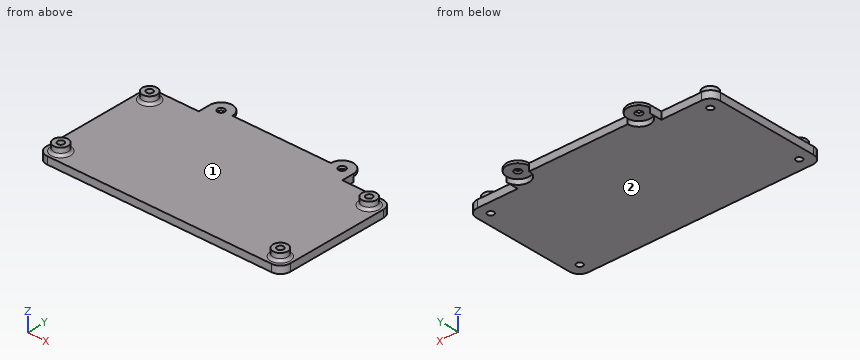
from build123d import *

# Parameters (mm, degrees)
SKETCH1_R           = 3
BOSS_EXTRUDE1_DEPTH = 3
SKETCH1_3_R         = 3
SKETCH1_3_R_2       = 1.3
BOSS_EXTRUDE2_DEPTH = 6
FILLET1_R           = 1
SKETCH2_R           = 1.4224
BOSS_EXTRUDE3_DEPTH = 3
CUT_EXTRUDE1_START  = -2
SKETCH6_R           = 4.618405104
CUT_EXTRUDE1_DEPTH  = 2


with BuildPart() as part:
    # Sketch1 → Boss-Extrude1 (new body)
    with BuildSketch(Plane.XY):
        with BuildLine():
            ThreePointArc((99.987500635, 4.00000762), (98.819645279, 1.180555381), (96.00019304, 0.012700025))
            Line((96.00019304, 0.012700025), (4.00000762, 0.012700025))
            ThreePointArc((4.00000762, 0.012700025), (1.180555381, 1.180555381), (0.012700025, 4.00000762))
            Line((0.012700025, 4.00000762), (0.012700025, 46.00009144))
            ThreePointArc((0.012700025, 46.00009144), (1.180555381, 48.819543679), (4.00000762, 49.987399035))
            Line((4.00000762, 49.987399035), (96.00019304, 49.987399035))
            ThreePointArc((96.00019304, 49.987399035), (98.819645279, 48.819543679), (99.987500635, 46.00009144))
            Line((99.987500635, 46.00009144), (99.987500635, 4.00000762))
        make_face()
        with Locations((95.0001905, 5.00001016)):
            Circle(SKETCH1_R, mode=Mode.SUBTRACT)
        with Locations((5.00001016, 5.00001016)):
            Circle(SKETCH1_R, mode=Mode.SUBTRACT)
        with Locations((95.0001905, 45.0000889)):
            Circle(SKETCH1_R, mode=Mode.SUBTRACT)
        with Locations((5.00001016, 45.0000889)):
            Circle(SKETCH1_R, mode=Mode.SUBTRACT)
    extrude(amount=BOSS_EXTRUDE1_DEPTH)

    # Sketch1<3> → Boss-Extrude2 (add)
    # profile 1 of 4: a face of its own
    with BuildSketch(Plane.XY):
        with Locations((5.00001016, 45.0000889)):
            Circle(SKETCH1_3_R)
        with Locations((5.00001016, 45.0000889)):
            Circle(SKETCH1_3_R_2, mode=Mode.SUBTRACT)
    # profile 2 of 4: a face of its own
    with BuildSketch(Plane.XY):
        with Locations((95.0001905, 45.0000889)):
            Circle(SKETCH1_3_R)
        with Locations((95.0001905, 45.0000889)):
            Circle(SKETCH1_3_R_2, mode=Mode.SUBTRACT)
    # profile 3 of 4: a face of its own
    with BuildSketch(Plane.XY):
        with Locations((95.0001905, 5.00001016)):
            Circle(SKETCH1_3_R)
        with Locations((95.0001905, 5.00001016)):
            Circle(SKETCH1_3_R_2, mode=Mode.SUBTRACT)
    # profile 4 of 4: a face of its own
    with BuildSketch(Plane.XY):
        with Locations((5.00001016, 5.00001016)):
            Circle(SKETCH1_3_R)
        with Locations((5.00001016, 5.00001016)):
            Circle(SKETCH1_3_R_2, mode=Mode.SUBTRACT)
    extrude(amount=BOSS_EXTRUDE2_DEPTH)

    # Fillet1
    fillet1_edges = [part.edges().sort_by_distance(p)[0] for p in [
        (92.0001905, 5.00001016, 3),
        (2.00001016, 5.00001016, 3),
        (92.0001905, 45.0000889, 3),
        (2.00001016, 45.0000889, 3),
    ]]
    fillet(fillet1_edges, radius=FILLET1_R)

    # Sketch2 → Boss-Extrude3 (add)
    with BuildSketch(Plane.XY.offset(3)):
        with BuildLine():
            Line((70.197495225, 54.987399035), (29.802705435, 54.987399035))
            ThreePointArc((29.802705434, 54.987399035), (25.18430033, 59.605804139), (20.565895226, 54.987399035))
            Line((20.565895225, 54.987399035), (20.565895225, 49.987399035))
            Line((20.565895225, 49.987399035), (79.434305435, 49.987399035))
            Line((79.434305435, 49.987399035), (79.434305435, 54.987399035))
            ThreePointArc((79.434305434, 54.987399035), (74.81590033, 59.605804139), (70.197495226, 54.987399035))
        make_face()
        with Locations((25.18430033, 54.987399035)):
            Circle(SKETCH2_R, mode=Mode.SUBTRACT)
        with Locations((74.81590033, 54.987399035)):
            Circle(SKETCH2_R, mode=Mode.SUBTRACT)
    extrude(amount=-BOSS_EXTRUDE3_DEPTH)

    # Sketch6 → Cut-Extrude1 (cut)
    with BuildSketch(Plane(origin=(0, 0, 0), x_dir=(-1, 0, 0), z_dir=(0, 0, -1)).offset(CUT_EXTRUDE1_START)):
        with Locations((-74.81590033, 54.987399035)):
            Circle(SKETCH6_R)
        with Locations((-25.18430033, 54.987399035)):
            Circle(SKETCH6_R)
    extrude(amount=CUT_EXTRUDE1_DEPTH, mode=Mode.SUBTRACT)


solid = part.part
Geometry check sheet. Reference: the model listing, model coordinates, mm. Face numbers are marked on the shaded views. Coordinates: 2 decimals unless noted, no trailing zeros. Order: outer loops, then holes, each group sorted by start corner. A loop starts at its lowest first (then second) coordinate and runs counter-clockwise, first axis right, second up. Notation, with made-up numbers: (-34.5, 38.25) - (-19.5, 38.25) arc R13 ccw to (-19.5, 48.25) - close; hole circle Ø6 at (16, 24). An arc over 180 degrees is marked (long way). Answer in a Markdown table with one row per item. Add a question column.
1) Cross-section at B-B, the plane x = 88.5. Record the cut outline in (y, z).
2) Cross-section at C-C, the plane y = 23.5. Record the cut outline in (x, z).
3) Cross-section at A-A, the plane z = 1.05. Record the cut outline in (x, y), then the cut area to 3 significant figures.
4) Gauge pin test, flat ends, axial feed: P1, Ø2.5, axis at y = 51.5, z = 1.5, coming from the +X side; P2, Ø2.5, axis at x = 55.5, z = 2, coming from the +Y side; P3, Ø3.5, axis at x = 88.5, z = 1.5, coming from the +Y side. Record the tip position at first contact, or that the pin passes through.
5) Material ranges on line 1 along Y through (x, z) = (96, 3.25); line 2 along Z through (x, y) = (57, 27.5); line 3 along X through (y, z) = (56.5, 2.4), recorded low to high. Write a range as [from, to].
6) Release check for a two-part mould opening along X. For the marked faces 1 and 2 record: +X half, -X half, draft (parallel to the pull), parting line (faces both ways), or undercut.
Check result:
| question | item | result |
|---|---|---|
| 1 | outline | (0.01, 0) - (49.99, 0) - (49.99, 3) - (0.01, 3) - close |
| 2 | outline | (0.01, 0) - (99.99, 0) - (99.99, 3) - (0.01, 3) - close |
| 3 | outline | (0.01, 4) arc R3.99 ccw to (4, 0.01) - (96, 0.01) arc R3.99 ccw to (99.99, 4) - (99.99, 46) arc R3.99 ccw to (96, 49.99) - (79.43, 49.99) - (79.43, 54.99) arc R4.62 cw to (70.2, 54.99) - (29.8, 54.99) arc R4.62 cw to (20.57, 54.99) - (20.57, 49.99) - (4, 49.99) arc R3.99 ccw to (0.01, 46) - close; hole circle Ø2.6 at (5, 5); hole circle Ø2.6 at (5, 45); hole circle Ø2.6 at (95, 5); hole circle Ø2.6 at (95, 45) |
| 3 | area | 5,190 mm² |
| 4 | P1 | stops at x = 79.43 |
| 4 | P2 | stops at y = 54.99 |
| 4 | P3 | stops at y = 49.99 |
| 5 | line 1 | y = [1.81, 4.17], [5.83, 8.19], [41.81, 44.17], [45.83, 48.19] |
| 5 | line 2 | z = [0, 3] |
| 5 | line 3 | x = [20.82, 29.55], [70.45, 79.18] |
| 6 | face 1 | undercut |
| 6 | face 2 | draft |
